```python
from build123d import *

# Parameters (mm, degrees)
SALIENTE_EXTRUIR2_DEPTH  = 100
SALIENTE_EXTRUIR3_DEPTH  = 200
CROQUIS11_W              = 37
CROQUIS11_H              = 37
CORTAR_EXTRUIR2_DEPTH    = 168.630546142
CROQUIS13_W              = 126.669935474
CROQUIS13_H              = 37
SALIENTE_EXTRUIR9_DEPTH  = 3
CROQUIS14_W              = 100
CROQUIS14_H              = 1.54
SALIENTE_EXTRUIR12_DEPTH = 50
SALIENTE_EXTRUIR13_REACH = 194.026
CROQUIS20_W              = 99.969357698
CROQUIS20_H              = 1.54
SALIENTE_EXTRUIR14_REACH = 152.336
CROQUIS21_W              = 100
CROQUIS21_H              = 1.54
CROQUIS22_W              = 25
CROQUIS22_H              = 1.45
SALIENTE_EXTRUIR15_DEPTH = 25
CROQUIS23_R              = 9.5
CORTAR_EXTRUIR9_DEPTH    = 1.45
CROQUIS24_R              = 12.5
CORTAR_EXTRUIR10_DEPTH   = 12.5


with BuildPart() as part:
    # Croquis5 → Saliente-Extruir2 (new, symmetric)
    with BuildSketch(Plane(origin=(0, 0, 0), x_dir=(0, 0, -1), z_dir=(1, 0, 0))):
        Polygon((-77.476042657, 3), (-88.67219508, 0), (100, 0), (100, 3), align=None)
    extrude(amount=SALIENTE_EXTRUIR2_DEPTH, both=True)

    # Croquis6 → Saliente-Extruir3 (add)
    with BuildSketch(Plane(origin=(100, 0, 0), x_dir=(0, 0, -1), z_dir=(1, 0, 0))):
        Polygon((-68.776042657, 3), (-16.81451843, 93), (-15.036279601, 93), (-66.997803828, 3), align=None)
    extrude(amount=-SALIENTE_EXTRUIR3_DEPTH)

    # Croquis11 → Cortar-Extruir2 (cut, through all)
    with BuildSketch(Plane(origin=(0, 3, 0), x_dir=(1, 0, 0), z_dir=(0, 1, 0))):
        with Locations((81.5, -18.5)):
            Rectangle(CROQUIS11_W, CROQUIS11_H)
        with Locations((-82.169935474, -18.5)):
            Rectangle(CROQUIS11_W, CROQUIS11_H)
    extrude(amount=-CORTAR_EXTRUIR2_DEPTH, mode=Mode.SUBTRACT)

    # Croquis13 → Saliente-Extruir9 (add)
    with BuildSketch(Plane(origin=(0, 3, 0), x_dir=(1, 0, 0), z_dir=(0, 1, 0))):
        with Locations((-0.334967737, -18.5)):
            Rectangle(CROQUIS13_W, CROQUIS13_H)
    extrude(amount=SALIENTE_EXTRUIR9_DEPTH)



with BuildPart() as body_2:
    # Croquis14 → Saliente-Extruir12 (new body)
    with BuildSketch(Plane.XY.offset(35)):
        with Locations((0, 51.77)):
            Rectangle(CROQUIS14_W, CROQUIS14_H)
    extrude(amount=-SALIENTE_EXTRUIR12_DEPTH)


with BuildPart() as part_1:
    add(part.part)

    add(body_2.part)  # Saliente-Extruir13 merges body 2
    # Saliente-Extruir13: up to this plane
    saliente_extruir13_end = Plane(origin=(-100, 93, 15.036279601), z_dir=(0, -0.4999999999999976, -0.86602540378444))
    # Croquis20 → Saliente-Extruir13 (add, up to the surface)
    with BuildSketch(Plane.XY.offset(35), mode=Mode.PRIVATE) as saliente_extruir13_sk1:
        with Locations((0.015321151, 51.77)):
            Rectangle(CROQUIS20_W, CROQUIS20_H)
    saliente_extruir13_tool1 = split(extrude(saliente_extruir13_sk1.sketch, amount=SALIENTE_EXTRUIR13_REACH, mode=Mode.PRIVATE), bisect_by=saliente_extruir13_end, keep=Keep.BOTH, mode=Mode.PRIVATE)
    add(saliente_extruir13_tool1.solids().sort_by_distance((0.015321, 51.77, 35))[0])

    # Croquis21 → Saliente-Extruir14 (add, up to next)
    with BuildSketch(Plane.XZ.offset(-51), mode=Mode.PRIVATE) as saliente_extruir14_sk1:
        with Locations((0, -14.23)):
            Rectangle(CROQUIS21_W, CROQUIS21_H)
    saliente_extruir14_tool1 = extrude(saliente_extruir14_sk1.sketch, amount=SALIENTE_EXTRUIR14_REACH, mode=Mode.PRIVATE) - part_1.part
    add(saliente_extruir14_tool1.solids().sort_by_distance((0, 51, -14.23))[0])

    # Croquis22 → Saliente-Extruir15 (add)
    with BuildSketch(Plane(origin=(0, 52.54, 0), x_dir=(1, 0, 0), z_dir=(0, 1, 0))):
        with Locations((0, -10.725)):
            Rectangle(CROQUIS22_W, CROQUIS22_H)
    extrude(amount=SALIENTE_EXTRUIR15_DEPTH)

    # Croquis23 → Cortar-Extruir9 (cut)
    with BuildSketch(Plane(origin=(0, 0, 10), x_dir=(-1, 0, 0), z_dir=(0, 0, -1))):
        with Locations((0, 65.54)):
            Circle(CROQUIS23_R)
    extrude(amount=-CORTAR_EXTRUIR9_DEPTH, mode=Mode.SUBTRACT)

    # Croquis24 → Cortar-Extruir10 (cut, symmetric)
    with BuildSketch(Plane.XY.offset(35)):
        with Locations(Location((0, 65.54, 0), (0, 0, 270))):
            Circle(CROQUIS24_R)
    extrude(amount=CORTAR_EXTRUIR10_DEPTH, both=True, mode=Mode.SUBTRACT)


solid = part_1.part
```
Design review of the part built by this model. Coordinates are the model's own, in mm. A direction names the side the tool comes from. Give positions to 0.01 mm unless a question says otherwise; leave off trailing zeros. Loops run counter-clockwise (first coordinate to the right, second up) from the corner with the lowest first, then second, coordinate; pieces in that order, holes last. Notation, with made-up numbers: (-29.5, 23) -> (-13.5, 23) arc R4 ccw to (-13.5, 27) -> close; hole circle Ø8 at (40, -6). An arc over 180 degrees is marked (long way). Write each question's results on one line, items separated by ' | '.
Q1. Take a section at D-D, the plane x = 59. Write out the cut boundary in (y, z), plus the area to 3 significant figures.
Reply:
outline: (0, -100) -> (3, -100) -> (3, 0) -> (6, 0) -> (6, 37) -> (3, 37) -> (3, 67) -> (93, 15.04) -> (93, 16.81) -> (3, 68.78) -> (3, 77.48) -> (0, 88.67) -> close | area: 820 mm²
Q2. Take a section at A-A, the plane z = -11. Write out the cut boundary in (x, y).
Reply:
outline: (-100, 0) -> (100, 0) -> (100, 3) -> (-100, 3) -> close; (-50, 51) -> (50, 51) -> (50, 52.54) -> (-50, 52.54) -> close
Q3. Take a section at B-B, the plane x = 19.5. Write out the cut boundary in (y, z) (3 decimals).
Reply:
outline: (0, -100) -> (3, -100) -> (3, -15) -> (52.54, -15) -> (52.54, 38.396) -> (93, 15.036) -> (93, 16.815) -> (3, 68.776) -> (3, 77.476) -> (0, 88.672) -> close; hole (3, -13.46) -> (51, -13.46) -> (51, 39.285) -> (3, 66.998) -> (3, 37) -> (6, 37) -> (6, 0) -> (3, 0) -> close
Q4. The part is to be moulded in two halves that separate along Z. For faces 1 (the face through (1, 0, -4)), 2 (the face through (-1, 27, -13.46)), 3 (the face through (-6, 57, 10)), say which applies: +Z half, -Z half, draft (parallel to the pull), parting line (faces both ways), or undercut.
Reply:
face 1: draft | face 2: undercut | face 3: -Z half
Q5. Machinability: for faces 4 (the face through (-63.67, 3, 19)), 5 (the face through (-6, 57, 11.45)), 6 (the face through (12.467, 64.63, 31.668)), 7 (the face through (63, 3, 19)), 8 (the face through (1, 3, 52)), which of the approach directions +Z, -Z, +X, -X, +Y, -Y give a long, thin tool a straight path to every point of the face, cutting with its end or side? Answer none if there is none.
Reply:
face 4: -X, -Y | face 5: +X, -X, +Y | face 6: +Z | face 7: +X, -Y | face 8: +X, -X
Q6. Take a section at C-C, the plane y = 70. Write out the cut boundary in (x, z), plus the area to 3 significant figures.
Reply:
outline: (-100, 28.32) -> (-11.68, 28.32) -> (-11.68, 30.09) -> (-100, 30.09) -> close; (-12.5, 10) -> (-8.39, 10) -> (-8.39, 11.45) -> (-12.5, 11.45) -> close; (8.39, 10) -> (12.5, 10) -> (12.5, 11.45) -> (8.39, 11.45) -> close; (11.68, 28.32) -> (100, 28.32) -> (100, 30.09) -> (11.68, 30.09) -> close | area: 326 mm²
Q7. Wall thickness on L1, parallel to Y at x = 0, z = 10.85; L2, parallel to X at y = 36, z = -14.5; L3, parallel to Y at x = 8, z = 22: over which ranges is each line inside the solid? List them lowest first.
Reply:
L1: y = 0 to 6, 51 to 56.04, 75.04 to 77.54 | L2: x = -50 to 50 | L3: y = 0 to 6, 51 to 52.54, 80.94 to 84.02
Q8. For pin 1 Ø0.7 at (x, z) = (-3, 10.5) entering from +Y; pin 2 Ø5 at (x, z) = (21.5, -75) entering from -Y; pin 3 Ø5 at (y, z) = (4, 24.5) entering from +X; pin 4 Ø3 at (x, y) = (-25.5, 74.5) entering from +Z, all flat-tipped, find the tip position at first contact; note any pin that passes through.
Reply:
pin 1: stops at y = 77.54 | pin 2: stops at y = 0 | pin 3: stops at x = 63 | pin 4: stops at z = 28.36
